The listing builds one solid part. Answer for the finished solid, in the listing's coordinates (mm). Face numbers are marked on the shaded views. A direction names the side the tool comes from. Give positions to 0.01 mm unless a question says otherwise; leave off trailing zeros. Order: outer loops, then holes, each group sorted by start corner. A loop starts at its lowest first (then second) coordinate and runs counter-clockwise, first axis right, second up. Notation, with made-up numbers: (11.25, 5) - (63.25, 5) arc R26 cw to (63.25, 32) - close; hole circle Ø7 at (67.5, 19). An arc over 180 degrees is marked (long way). Use CSV: the item, a comma, the result in double quotes.
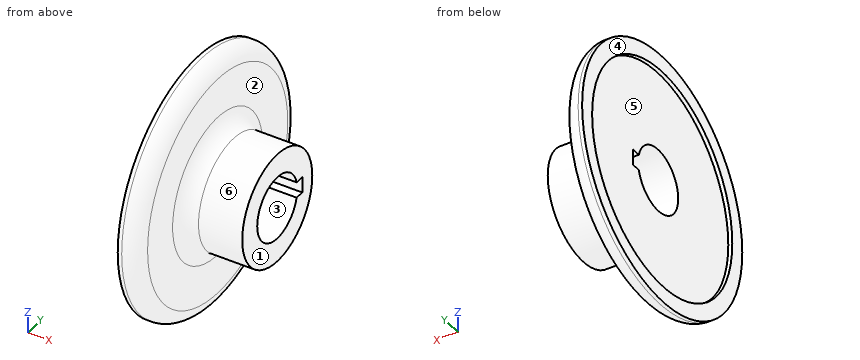
Autodesk Inventor part; units mm, degrees
ref_plane "YZ Plane" through (0, 0, 0) normal (1, 0, 0) x (0, 1, 0)
ref_plane "XZ Plane" through (0, 0, 0) normal (0, 1, 0) x (-1, 0, 0)
ref_plane "XY Plane" through (0, 0, 0) normal (0, 0, 1) x (1, 0, 0)
sketch "Sketch1" plane through (0, 0, 0) normal (0, 0, 1) x (1, 0, 0)
  line L0 (0, 25.4) -> (0.7937, 25.4)
  line L1 (3.9687, 22.225) -> (3.9688, 14.2875)
  line L2 (7.1437, 11.1125) -> (15.875, 11.1125)
  line L3 (0, 25.4) -> (0, 22.225)
  line L4 (-3.175, 0) -> (19.05, 0)
  line L5 (0, -5.2115) -> (0, 31.2691) construction
  line L6 (15.875, 11.1125) -> (15.875, 6.35)
  arc A0 (3.9687, 22.225) -> (0.7937, 25.4) centre (0.7937, 22.225) ccw
  arc A1 (3.9688, 14.2875) -> (7.1437, 11.1125) centre (7.1438, 14.2875) ccw
  line L7 (0.7937, 22.225) -> (0.7937, 6.35)
  line L8 (0.7937, 22.225) -> (0, 22.225)
  line L9 (0.7937, 6.35) -> (15.875, 6.35)
  point P0 (0, 0)
  dimension "d0" = 50.8
  dimension "d1" = 22.225
  dimension "d2" = 0
  dimension "d3" = 15.875
  dimension "d4" = 3.9688
  dimension "d5" = 3.175
  dimension "d6" = 0.7937
  dimension "d7" = 44.45
  dimension "d8" = 12.7
revolve "Revolution1" add sketch "Sketch1" angle 360 about axis through (-10, 0, 0) along (1, 0, 0)
sketch "Sketch2" plane through (15.875, 0, 0) normal (1, 0, 0) x (0, 0, -1)
  line L0 (0, -35.56) -> (0, 35.56) construction
  line L1 (35.56, 0) -> (-35.56, 0) construction
  line L2 (-1.5875, 7.9375) -> (1.5875, 7.9375)
  line L3 (1.5875, 7.9375) -> (1.5875, 4.7625)
  line L4 (1.5875, 4.7625) -> (-1.5875, 4.7625)
  line L5 (-1.5875, 4.7625) -> (-1.5875, 7.9375)
  line L6 (-4.6004, 6.35) -> (6.3294, 6.35) construction
  circle A0 centre (0, 0) radius 6.35 construction
  dimension "d10" = 3.175
  dimension "d11" = 1.5875
  dimension "d12" = 1.5875
  dimension "d13" = 3.175
extrude "Extrusion1" cut sketch "Sketch2" against normal through all
equation "\"d11\" = 0.5 * d10"
equation "\"d13\" = 2 * d12"
properties part number "Brida de la Rueda" material "Aluminum 6061-AHC"
Item 1: The part is cut by section D-D (x = 4.75). Give the vertices of the cut face in (y, z), and give its area (3 significant figures).
Taken from the geometry:
outline,"circle Ø24.4 at (0, 0); hole (6.15, -1.59) - (7.94, -1.59) - (7.94, 1.59) - (6.15, 1.59) arc R6.35 ccw (long way) to start"
area,"336 mm^2"
Item 2: Find the intervals of material crossed by line 1 along Z through (x, y) = (0.45, 0) (3 decimals); line 2 along Z through (x, y) = (12, 0); line 3 along X through (y, z) = (15, 9), in increasing order.
Taken from the geometry:
line 1,"-25.4 to -22.225, 22.225 to 25.4"
line 2,"-11.11 to -6.35, 6.35 to 11.11"
line 3,"0.79 to 3.97"
Item 3: The mould has two halves that part along Z. Classify the marked faces 3, 4, 5 and 6: +Z half, -Z half, draft (parallel to the pull), parting line (faces both ways), or undercut.
Taken from the geometry:
face 3,"undercut"
face 4,"draft"
face 5,"undercut"
face 6,"parting line"
Item 4: Each of these flat-tipped pins is pushed along its axis until it touches: pin 1 (1 mm diameter, centred on x = 6.5, z = -0.5, fed in from -Y); pin 2 (10 mm diameter, centred on y = -0.5, z = -10, fed in from -X); pin 3 (1.4 mm diameter, centred on x = 11.5, y = 7, fed in from +Z); pin 4 (8 mm diameter, centred on y = -1, z = -14.5, fed in from +X) (3 decimals). Where does it stop, or does it pass through?
Taken from the geometry:
pin 1,"y = -11.32"
pin 2,"x = 0.79"
pin 3,"z = 9.15"
pin 4,"x = 15.875"
Item 5: Which of the six approach directions +Z, -Z, +X, -X, +Y, -Y give full straight-line access (tool end or side, diameter ignored) to the marked faces 1 and 2?
Taken from the geometry:
face 1,"+Z, -Z, +X, +Y, -Y"
face 2,"+X"
